Could you check a few things on this model? Use its own coordinates, in mm. A direction names the side the tool comes from. Round coordinates to 2 decimals unless told otherwise and drop trailing zeros. Loops run counter-clockwise (first coordinate to the right, second up) from the corner with the lowest first, then second, coordinate; pieces in that order, holes last. Notation, with made-up numbers: M 55,-5.5 L 105,-5.5 A10 ccw 105,1.5 Z; hole C -37,72 d11. An arc over 180 degrees is marked long. One line per item, written item: value. Start each with the question number.
Q1. Please list where these lines run through material, in increasing order: line 1 along Y through (x, z) = (-0.25, -20.5); line 2 along Y through (x, z) = (0, -35); line 3 along Z through (x, y) = (-4, 3).
Q2. Imagine slicing it at D-D (z = -40). Please give me the cut outline in (x, y).
Q3. Imagine slicing it at A-A (x = 0). Please give me the cut outline in (y, z) (3 decimals).
Q4. I'm going to push flat-ended pins straight in: pin 1 Ø1.5 at (y, z) = (-2.5, -30) entering from -X; pin 2 Ø1.5 at (x, y) = (1.5, 0) entering from +Z; pin 3 Ø2 at (x, z) = (-10, -37.5) entering from +Y. Where does each tip first touch, or does it pass through?
Q5. Imagine slicing it at B-B (z = -7). Please give me the cut outline in (x, y) (3 decimals), then the cut area to 3 significant figures.
Q6. Thinking about a two-plate mould opening in X: for faces 1 (the face through (-0.69, -3.1, -12.32)), 2 (the face through (-10.1, 7.7, -34.3)), 3 (the face through (0, 0, -28.6)), 4 (the face through (3, -6, -53.6)), which applies, released by +X, released by -X, zero draft, split by the parting line, or undercut?
Q7. Which directions (+Z, -Z, +X, -X, +Y, -Y) give clear straight access to the entire face, cutting with the end or side of a thin tool? Please do faces 5 (the face through (2.93, 5.634, -41.275)), 6 (the face through (2, -3, 0)), 7 (the face through (-3, -6, -14.4)).
from build123d import *

# Parameters (mm, degrees)
SKETCH2_R          = 3.175
CUT_EXTRUDE1_DEPTH = 25
SKETCH3_R          = 6.35
CUT_EXTRUDE2_DEPTH = 25


with BuildPart() as part:
    # Sketch1 → Revolve1 (revolve)
    with BuildSketch(Plane(origin=(0, 0, 0), x_dir=(0, 0, -1), z_dir=(1, 0, 0)), mode=Mode.PRIVATE) as revolve1_sk:
        Polygon((14.4, 6.35), (14.4, 12.7), (53.6, 12.7), (53.6, 0), (0, 0), (0, 6.35), align=None)
    revolve(revolve1_sk.sketch.rotate(Axis((0, 0, 0), (0, 0, -1)), 90), axis=Axis((0, 0, 0), (0, 0, -1)))

    # Sketch2 → Cut-Extrude1 (cut)
    with BuildSketch(Plane.XY):
        Circle(SKETCH2_R)
    extrude(amount=-CUT_EXTRUDE1_DEPTH, mode=Mode.SUBTRACT)

    # Sketch3 → Cut-Extrude2 (cut)
    with BuildSketch(Plane(origin=(0, 0, -53.6), x_dir=(-1, 0, 0), z_dir=(0, 0, -1))):
        with Locations(Location((0, 0, 0), (0, 0, 180))):
            Circle(SKETCH3_R)
    extrude(amount=-CUT_EXTRUDE2_DEPTH, mode=Mode.SUBTRACT)


solid = part.part
Report:
1. line 1: y = -12.7 to -3.17, 3.17 to 12.7
1. line 2: y = -12.7 to -6.35, 6.35 to 12.7
1. line 3: z = -28.6 to 0
2. outline: C 0,0 d25.4; hole C 0,0 d12.7
3. outline: M -12.7,-53.6 L -6.35,-53.6 L -6.35,-28.6 L 6.35,-28.6 L 6.35,-53.6 L 12.7,-53.6 L 12.7,-14.4 L 6.35,-14.4 L 6.35,0 L 3.175,0 L 3.175,-25 L -3.175,-25 L -3.175,0 L -6.35,0 L -6.35,-14.4 L -12.7,-14.4 Z
4. pin 1: stops at x = -12.58
4. pin 2: stops at z = -25
4. pin 3: stops at y = 8.96
5. outline: C 0,0 d12.7; hole C 0,0 d6.35
5. area: 95.0 mm²
6. face 1: undercut
6. face 2: split by the parting line
6. face 3: undercut
6. face 4: zero draft
7. face 5: -Z
7. face 6: +Z, +X, -X, +Y, -Y
7. face 7: +Z
